Geometry: see drawing. Coordinates: mm, zero at the bounding-box minimum. A direction names the side the tool comes from. Give positions to 0.01 mm unless a question says otherwise; leave off trailing zeros. Write each loop counter-clockwise with the first axis right and the second up, starting at its lowest first coordinate (ties: lowest second). Pieces come first, ordered by that corner, then holes. Notation, with made-up numbers: M 46.25,46 L 52.25,46 A9 ccw 52.25,51 Z; hole C 28.25,-39 d1. An arc over 180 degrees is marked long. Use a Markdown table: item, result. Add a question column.
1) Pin query (flat end, axial travel): pin 1 (4 mm diameter, centred on x = 5.5, y = 35.5, fed in from +Z); pin 2 (1 mm diameter, centred on y = 23, z = 5.5, fed in from -X); pin 3 (3 mm diameter, centred on y = 12, z = 4, fed in from -X). Return the tip coordinate at first contact, or that it passes through.
2) Section A-A on x = 4.25. Return the cut outline in (y, z), then the cut area to 3 significant figures.
3) Section B-B on z = 4.25. Return the cut outline in (x, y), then the cut area to 3 significant figures.
4) Section C-C on y = 11. Return the cut outline in (x, z), then the cut area to 3 significant figures.
5) Section D-D on y = 55. Return the cut outline in (x, z).
6) Set-up query: the marked faces 1 and 2. Return all of +Z, -Z, +X, -X, +Y, -Y with unobstructed straight access to the full face (end or side cutting, diameter ignored); none if empty.
7) Line query: line 1 (Y direction, x = 3.15, z = 4.25); line 2 (Z direction, x = 4, y = 55); line 3 (Z direction, x = 4, y = 20). Output: solid intervals per line, ascending.
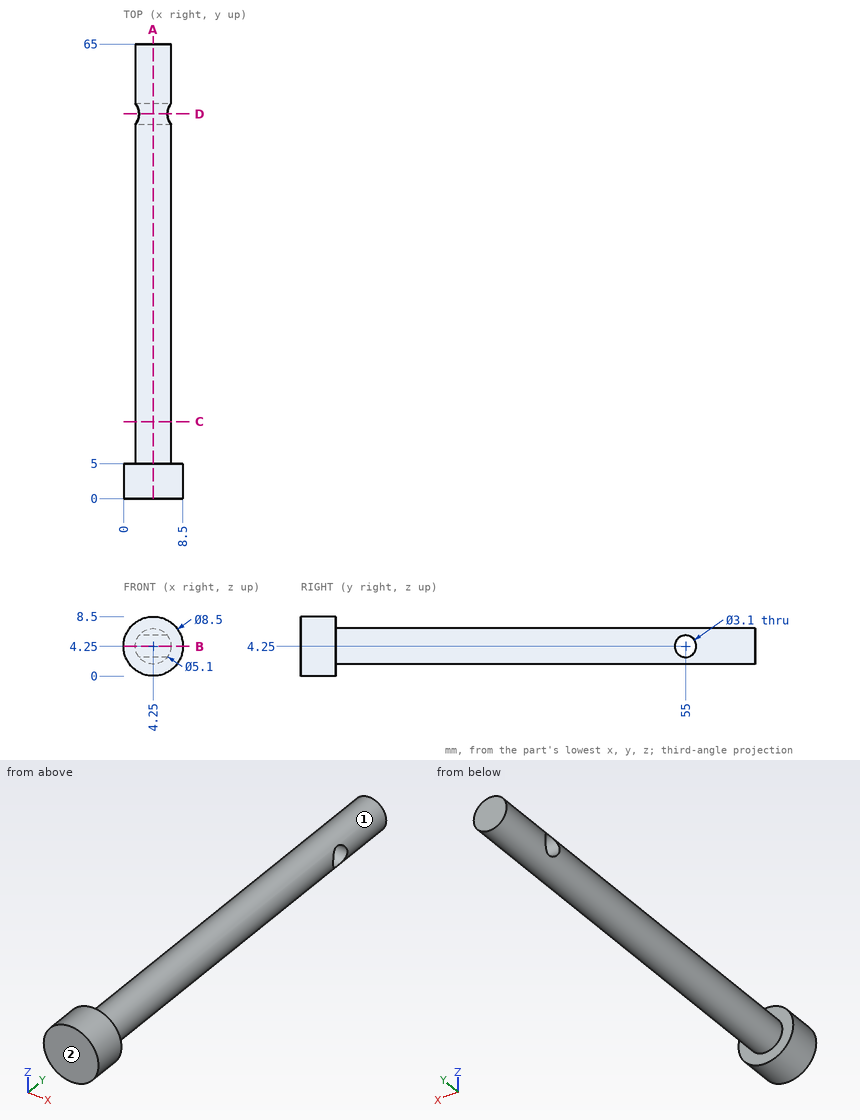
Found:
| question | item | result |
|---|---|---|
| 1 | pin 1 | z = 6.8 |
| 1 | pin 2 | x = 1.81 |
| 1 | pin 3 | x = 1.7 |
| 2 | outline | M 0,0 L 5,0 L 5,1.7 L 65,1.7 L 65,6.8 L 5,6.8 L 5,8.5 L 0,8.5 Z; hole C 55,4.25 d3.1 |
| 2 | area | 341 mm² |
| 3 | outline | M 0,0 L 8.5,0 L 8.5,5 L 6.8,5 L 6.8,53.45 L 1.7,53.45 L 1.7,5 L 0,5 Z; M 1.7,56.55 L 6.8,56.55 L 6.8,65 L 1.7,65 Z |
| 3 | area | 333 mm² |
| 4 | outline | C 4.25,4.25 d5.1 |
| 4 | area | 20.4 mm² |
| 5 | outline | M 2.23,2.7 A2.55 ccw 6.27,2.7 Z; M 2.23,5.8 L 6.27,5.8 A2.55 ccw Z |
| 6 | face 1 | +Y |
| 6 | face 2 | +Z, -Z, +X, -X, -Y |
| 7 | line 1 | 0 to 53.45, 56.55 to 65 |
| 7 | line 2 | 1.71 to 2.7, 5.8 to 6.79 |
| 7 | line 3 | 1.71 to 6.79 |
